Could you check a few things on this drawing? It's one solid part, dimensions in mm from its lowest x, y, z. A direction names the side the tool comes from. Round coordinates to 2 decimals unless told otherwise and drop trailing zeros. Loops run counter-clockwise (first coordinate to the right, second up) from the corner with the lowest first, then second, coordinate; pieces in that order, holes last. Notation, with made-up numbers: M 33,84.5 L 44,84.5 A19 ccw 44,88.5 Z; hole C 50,55 d4. An arc over 180 degrees is marked long. Answer as a JSON object with one key per item and string values.
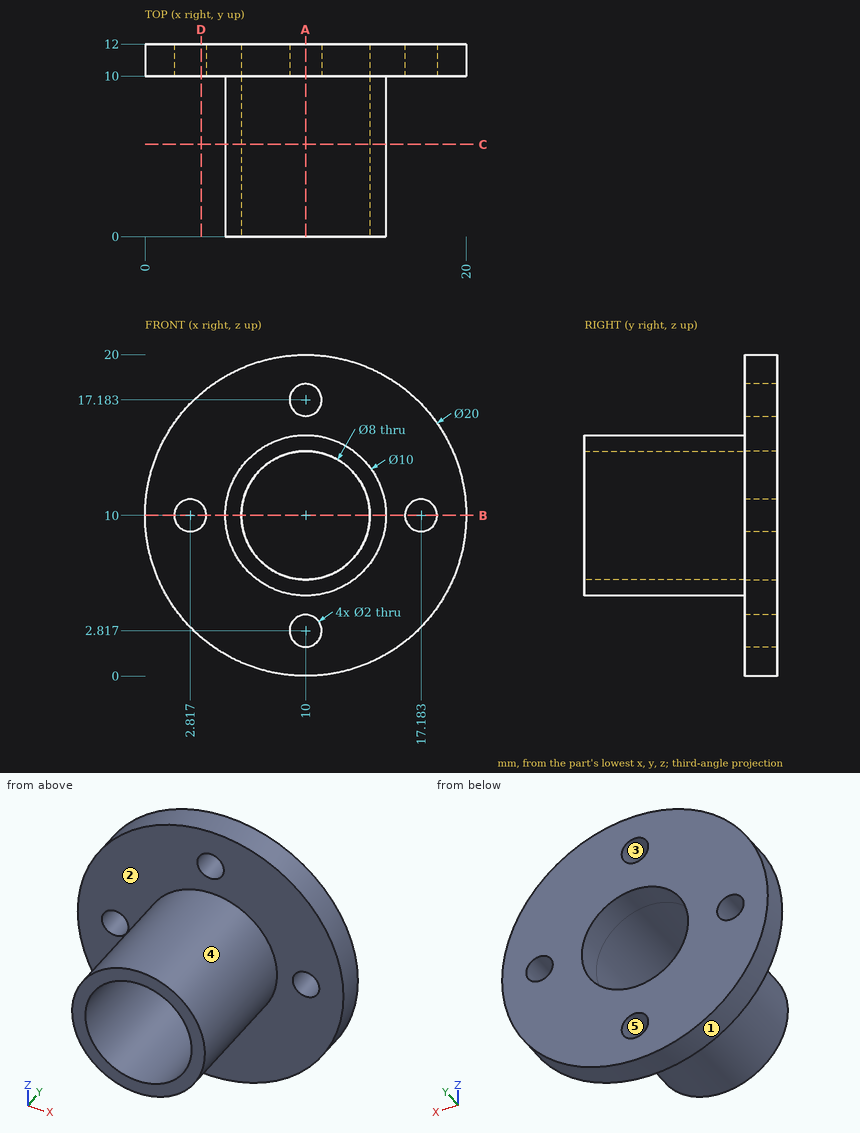
Item 1: On a 3-axis mill with a long thin cutter (end or side, diameter ignored), from which of +Z, -Z, +X, -X, +Y, -Y can I reach the whole of each face in a straight line? I mean the marked faces 4 and 5. Say none if no direction works.
Resolved:
{"face 4": "-Y", "face 5": "+Y, -Y"}
Item 2: Please list where these lines run through material, in increasing order: probe 1 along X at (y, z) = (10.55, 10); probe 2 along Y at (x, z) = (16.75, 5); probe 3 along X at (y, z) = (1.5, 9). Write a range as from..to.
Resolved:
{"probe 1": "0..1.82, 3.82..6, 14..16.18, 18.18..20", "probe 2": "10..12", "probe 3": "5.1..6.13, 13.87..14.9"}
Item 3: If we mould it in two halves opening along X, with no side actions, what happens to the marked faces 1, 2 and 3? For each: pulls with the +X half, pulls with the -X half, needs draft (parallel to the pull), parting line crosses it, or undercut.
Resolved:
{"face 1": "parting line crosses it", "face 2": "needs draft", "face 3": "undercut"}
Item 4: I want a section at B-B, the plane z = 10. Please give me the cut outline in (x, y).
Resolved:
{"outline": "M 0,10 L 1.82,10 L 1.82,12 L 0,12 Z; M 3.82,10 L 5,10 L 5,0 L 6,0 L 6,12 L 3.82,12 Z; M 14,0 L 15,0 L 15,10 L 16.18,10 L 16.18,12 L 14,12 Z; M 18.18,10 L 20,10 L 20,12 L 18.18,12 Z"}
Item 5: I want a section at A-A, the plane x = 10. Please give me the cut outline in (y, z).
Resolved:
{"outline": "M 0,5 L 10,5 L 10,3.82 L 12,3.82 L 12,6 L 0,6 Z; M 0,14 L 12,14 L 12,16.18 L 10,16.18 L 10,15 L 0,15 Z; M 10,0 L 12,0 L 12,1.82 L 10,1.82 Z; M 10,18.18 L 12,18.18 L 12,20 L 10,20 Z"}
Item 6: I want a section at C-C, the plane y = 5.75. Please give me the cut outline in (x, z).
Resolved:
{"outline": "C 10,10 d10; hole C 10,10 d8"}
Item 7: I want a section at D-D, the plane x = 3.5. Please give me the cut outline in (y, z).
Resolved:
{"outline": "M 10,2.4 L 12,2.4 L 12,9.27 L 10,9.27 Z; M 10,10.73 L 12,10.73 L 12,17.6 L 10,17.6 Z"}
Item 8: I'm going to push flat-ended pins straight in: pin 1 Ø6 at (x, y) = (5, 4.5) entering from +Z; pin 2 Ø1.5 at (x, y) = (7.5, 2) entering from +Z; pin 3 Ø1 at (y, z) = (7.5, 6) entering from -X; pin 4 Ø1.2 at (x, z) = (17.18, 10) entering from -Y. Where does each tip first touch, or does it pass through?
Resolved:
{"pin 1": "z = 14.58", "pin 2": "z = 14.68", "pin 3": "x = 6.43", "pin 4": "through"}
